Check sheet for the modelled part. Datum: model origin and axes. Units: mm. Round coordinates to 2 decimals unless told otherwise and drop trailing zeros. Order: outer loops, then holes, each group sorted by start corner. A loop starts at its lowest first (then second) coordinate and runs counter-clockwise, first axis right, second up.
(1) Sectioned sample at C-C, the plane y = 4.7. Enter the section's corners in (x, z).
(2) Sectioned sample at B-B, the plane z = -10. Enter the section's corners in (x, y).
(3) Thickness scan on probe 1 along X at (y, z) = (4.05, -10); probe 2 along Z at (x, y) = (108, 4.7); probe 3 along X at (y, z) = (0.4, -5). Record the ranges inside material, lowest first.
(4) Sectioned sample at A-A, the plane x = 108. Enter the section's corners in (y, z).
(5) Depth check by flat-ended pin: pin 1 (7.5 mm diameter, centred on x = 108, z = -10, fed in from -Y). Enter the tip coordinate at first touch or a pass-through.
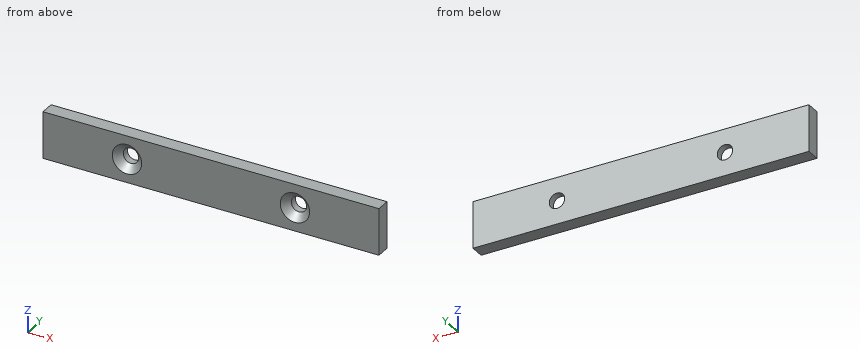
Autodesk Inventor part; units mm, degrees
ref_plane "YZ Plane" through (0, 0, 0) normal (1, 0, 0) x (0, 1, 0)
ref_plane "XZ Plane" through (0, 0, 0) normal (0, 1, 0) x (-1, 0, 0)
ref_plane "XY Plane" through (0, 0, 0) normal (0, 0, 1) x (1, 0, 0)
sketch "Sketch1" plane through (0, 0, 0) normal (0, 1, 0) x (-1, 0, 0)
  line L0 (0, 0) -> (-144, 0)
  line L1 (-144, 0) -> (-144, -20)
  line L2 (-144, -20) -> (0, -20)
  line L3 (0, -20) -> (0, 0)
  point P0 (-36, -10)
  point P1 (-108, -10)
  dimension "d0" = 144
  dimension "d1" = 20
extrude "Extrusion1" add sketch "Sketch1" along normal blind 6
hole "Hole1" at (36, 0, -10) at (108, 0, -10) direction (0, 1, 0) diameter 6.6 end through all countersink diameter 12.6 countersink angle 90
properties part number "chapa_base" material "Iron, Cast"
Derived:
1. outline: (0, -20) - (144, -20) - (144, 0) - (0, 0) - close; hole circle Ø6.6 at (36, -10); hole circle Ø6.6 at (108, -10)
2. outline: (0, 0) - (29.7, 0) - (32.7, 3) - (32.7, 6) - (0, 6) - close; (39.3, 3) - (42.3, 0) - (101.7, 0) - (104.7, 3) - (104.7, 6) - (39.3, 6) - close; (111.3, 3) - (114.3, 0) - (144, 0) - (144, 6) - (111.3, 6) - close
3. probe 1: x = 0 to 32.7, 39.3 to 104.7, 111.3 to 144
3. probe 2: z = -20 to -13.3, -6.7 to 0
3. probe 3: x = 0 to 32.87, 39.13 to 104.87, 111.13 to 144
4. outline: (0, -20) - (6, -20) - (6, -13.3) - (3, -13.3) - (0, -16.3) - close; (0, -3.7) - (3, -6.7) - (6, -6.7) - (6, 0) - (0, 0) - close
5. pin 1: stops at y = 2.55
